Autodesk Inventor part; units mm, degrees
ref_plane "YZ Plane" through (0, 0, 0) normal (1, 0, 0) x (0, 1, 0)
ref_plane "XZ Plane" through (0, 0, 0) normal (0, 1, 0) x (-1, 0, 0)
ref_plane "XY Plane" through (0, 0, 0) normal (0, 0, 1) x (1, 0, 0)
sketch "Skizze1" plane through (0, 0, 0) normal (0, 1, 0) x (-1, 0, 0)
  line L0 (-20.5, 20.5) -> (20.5, 20.5)
  line L1 (20.5, 20.5) -> (20.5, -20.5)
  line L2 (20.5, -20.5) -> (-20.5, -20.5)
  line L3 (-20.5, -20.5) -> (-20.5, 20.5)
  line L4 (-20.5, 20.5) -> (20.5, -20.5) construction
  line L5 (20.5, 20.5) -> (-20.5, -20.5) construction
  point P0 (0, 0)
  dimension "d0" = 41
  dimension "d1" = 41
extrude "Extrusion1" add sketch "Skizze1" along normal mid plane 39
sketch "Skizze2" plane through (0, -19.5, 0) normal (0, -1, 0) x (1, 0, 0)
  line L0 (-20.5, 20.5) -> (20.5, 20.5)
  line L1 (-7.5, 20.5) -> (7.5, 20.5)
  line L2 (7.5, 20.5) -> (7.5, 23.5)
  line L3 (7.5, 23.5) -> (-7.5, 23.5)
  line L4 (-7.5, 23.5) -> (-7.5, 20.5)
  line L5 (0, -29.3) -> (0, 32.3)
  point P0 (0, 0)
  dimension "d4" = 15
  dimension "d5" = 3
extrude "Extrusion2" add sketch "Skizze2" against normal blind 3
sketch "Skizze3" plane through (0, -19.5, 0) normal (0, -1, 0) x (1, 0, 0)
  line L0 (-15.5, -15.5) -> (15.5, -15.5)
  line L1 (15.5, -15.5) -> (15.5, 15.5)
  line L2 (15.5, 15.5) -> (-15.5, 15.5)
  line L3 (-15.5, 15.5) -> (-15.5, -15.5)
  line L4 (-15.5, -15.5) -> (15.5, 15.5) construction
  line L5 (15.5, -15.5) -> (-15.5, 15.5) construction
  circle A0 centre (-15.5, 15.5) radius 1.5
  circle A1 centre (15.5, 15.5) radius 1.5
  circle A2 centre (15.5, -15.5) radius 1.5
  circle A3 centre (-15.5, -15.5) radius 1.5
  circle A4 centre (0, 0) radius 4.5
  dimension "d8" = 31
  dimension "d9" = 31
  dimension "d10" = 3
  dimension "d11" = 9
extrude "Extrusion3" cut sketch "Skizze3" along normal through all both and the other way through all contours L3 A3 L0 | L0 A3 L3 | A2 L1 L0 | L0 L1 A2 | A0 L2 L3 | L3 L2 A0 | A1 L2 L1 | L1 L2 A1 | A4
chamfer "Fase1" distance 4 angle 45 4 edges at (20.5, 0, 20.5) (-20.5, 0, 20.5) (20.5, 0, -20.5) (-20.5, 0, -20.5)
sketch "Skizze4" plane through (0, 0, 0) normal (0, 1, 0) x (-1, 0, 0)
  line L0 (19.5, 14.6716) -> (14.6716, 19.5)
  line L1 (-14.6716, 19.5) -> (-19.5, 14.6716)
  line L2 (-19.5, -14.6716) -> (-14.6716, -19.5)
  line L3 (14.6716, -19.5) -> (19.5, -14.6716)
  line L4 (25.5, -25.5) -> (-25.5, -25.5)
  line L5 (-25.5, -25.5) -> (-25.5, 25.5)
  line L6 (-25.5, 25.5) -> (25.5, 25.5)
  line L7 (25.5, 25.5) -> (25.5, -25.5)
  line L8 (25.5, -25.5) -> (-25.5, 25.5) construction
  line L9 (-25.5, -25.5) -> (25.5, 25.5) construction
  line L10 (-20.5, 16.5) -> (-16.5, 20.5)
  line L11 (-16.5, -20.5) -> (-20.5, -16.5)
  line L12 (20.5, -16.5) -> (16.5, -20.5)
  line L13 (16.5, 20.5) -> (20.5, 16.5)
  line L14 (19.5, 14.6716) -> (19.5, -14.6716)
  line L15 (14.6716, -19.5) -> (-14.6716, -19.5)
  line L16 (-19.5, -14.6716) -> (-19.5, 14.6716)
  line L17 (-14.6716, 19.5) -> (14.6716, 19.5)
  line L18 (16.5, 20.5) -> (-16.5, 20.5)
  line L19 (-20.5, 16.5) -> (-20.5, -16.5)
  line L20 (-16.5, -20.5) -> (16.5, -20.5)
  line L21 (20.5, -16.5) -> (20.5, 16.5)
  point P0 (0, 0)
  dimension "d21" = 2
  dimension "d22" = 1
  dimension "d24" = 1
  dimension "d25" = 1
extrude "Extrusion4" cut sketch "Skizze4" along normal mid plane 22 contours L4 L5 L6 L7 | L10 L18 L13 L21 L12 L20 L11 L19
sketch "Skizze6" plane through (-7.5, -16.5, 20.5) normal (0, 0, 1) x (1, 0, 0)
  line L0 (0, 0) -> (15, 0)
  line L1 (15, 0) -> (15, 3)
  line L2 (15, 3) -> (0, 3)
  line L3 (0, 3) -> (0, 0)
  line L4 (15, -3) -> (15, 0)
  line L5 (0, -3) -> (0, 0)
  line L6 (0, 0) -> (15, 0)
  line L7 (2.5, 1) -> (3.5, 1)
  line L8 (3.5, 1) -> (3.5, 2)
  line L9 (3.5, 2) -> (2.5, 2)
  line L10 (2.5, 2) -> (2.5, 1)
  line L11 (2.5, 1) -> (3.5, 2) construction
  line L12 (3.5, 1) -> (2.5, 2) construction
  line L13 (5.5, 1) -> (6.5, 1)
  line L14 (6.5, 1) -> (6.5, 2)
  line L15 (6.5, 2) -> (5.5, 2)
  line L16 (5.5, 2) -> (5.5, 1)
  line L17 (5.5, 1) -> (6.5, 2) construction
  line L18 (6.5, 1) -> (5.5, 2) construction
  line L19 (8.5, 1) -> (9.5, 1)
  line L20 (9.5, 1) -> (9.5, 2)
  line L21 (9.5, 2) -> (8.5, 2)
  line L22 (8.5, 2) -> (8.5, 1)
  line L23 (8.5, 1) -> (9.5, 2) construction
  line L24 (9.5, 1) -> (8.5, 2) construction
  line L25 (11.5, 1) -> (12.5, 1)
  line L26 (12.5, 1) -> (12.5, 2)
  line L27 (12.5, 2) -> (11.5, 2)
  line L28 (11.5, 2) -> (11.5, 1)
  line L29 (11.5, 1) -> (12.5, 2) construction
  line L30 (12.5, 1) -> (11.5, 2) construction
  line L31 (7.5, -10.8) -> (7.5, 43.8)
  point P0 (7.5, 16.5)
  point P1 (3, 1.5)
  point P2 (6, 1.5)
  point P3 (9, 1.5)
  point P4 (12, 1.5)
  point P5 (12, 1.5)
  point P6 (15, 1.5)
  dimension "d29" = 3
  dimension "d30" = 3
  dimension "d31" = 3
  dimension "d32" = 1
  dimension "d33" = 1
extrude "Extrusion6" cut sketch "Skizze6" against normal blind 5
sketch "Skizze7" plane through (0, 0, 0) normal (1, 0, 0) x (0, 1, 0)
  line L0 (34.5, 0) -> (34.5, 2.5)
  line L1 (34.5, 2.5) -> (20.5, 2.5)
  line L2 (20.5, 2.5) -> (20.5, 7.5)
  line L3 (20.5, 7.5) -> (19.5, 7.5)
  line L4 (19.5, -16.5) -> (19.5, 16.5)
  line L5 (19.5, 0) -> (34.5, 0)
  line L6 (19.5, 0) -> (19.5, 7.5)
  line L7 (38.5419, 0) -> (33.7383, 0)
  point P0 (0, 0)
  dimension "d37" = 5
  dimension "d38" = 1
  dimension "d39" = 15
  dimension "d40" = 15
revolve "Umdrehung1" add sketch "Skizze7" angle 360 about axis through (0, 19.5, 0) along (0, 1, 0)
equation "\"d24\" = d22"
equation "\"d25\" = d22"
equation "\"d33\" = d32"
properties part number "MotorBlock"
Source: CAD feature listing. Evaluate the final solid. Frame: model axes, mm. A direction names the side the tool comes from. Round coordinates to 2 decimals unless told otherwise and drop trailing zeros. Loops run counter-clockwise (first coordinate to the right, second up) from the corner with the lowest first, then second, coordinate; pieces in that order, holes last. Notation, with made-up numbers: M 23.5,83 L 27.5,83 A7 ccw 27.5,94 Z; hole C -34.75,37 d4. An arc over 180 degrees is marked long. Use a Markdown table: item, result. Add a question column.
1. Contact query for flat-ended pins moving along their axis: pin 1 (9.5 mm diameter, centred on x = 5, y = 17, fed in from +Z); pin 2 (1.5 mm diameter, centred on y = -18, z = 22.5, fed in from +X); pin 3 (1.5 mm diameter, centred on y = 20.5, z = -12.5, fed in from +X); pin 4 (1.5 mm diameter, centred on x = 13.5, y = 3.5, fed in from -Z). Output: stop coordinate, or through.
2. Cut plane B-B, the plane x = -10. Output: boundary loops of the cut face in (y, z), and give its area (4 significant figures).
3. Cut plane A-A, the plane y = 16.5. Output: boundary loops of the cut face in (x, z).
4. Cut plane C-C, the plane z = -8.5. Output: boundary loops of the cut face in (x, y), and give its area (4 significant figures).
5. Ray query, line 1 along Y through (x, z) = (-7, 20); line 2 along Z through (x, y) = (-15, 10); line 3 along Z through (x, y) = (0, -9.5). Return the intervals inside material, ascending. Write a range as [from, to].
6. Set-up query: faces 1 (the flat face through (17.12, 0.15, -17.05)), 2 (the flat face through (-17.05, 0.15, -17.12)), 3 (the flat face through (2, 20.5, -2)), 4 (the flat face through (0, -13.5, 18)), 5 (the flat face through (0, 0, 19.5)). Return all of +Z, -Z, +X, -X, +Y, -Y with unobstructed straight access to the full face (end or side cutting, diameter ignored); none if empty.
7. Pull-direction query (X, two-part tool) for faces 6 (the flat face through (0, 19.5, -9)), 7 (the flat face through (-7.5, -18, 22)), 8 (the flat face through (20.5, -15, 0)), 9 (the flat face through (7.5, -15, 18)); classes: +X half, -X half, draft (parallel to the pull), parting line (faces both ways), or undercut.
8. Cut plane D-D, the plane x = -15.5. Output: boundary loops of the cut face in (y, z), and give its area (3 significant figures).
Solution:
| question | item | result |
|---|---|---|
| 1 | pin 1 | stops at z = 20.5 |
| 1 | pin 2 | stops at x = 7.5 |
| 1 | pin 3 | passes through |
| 1 | pin 4 | stops at z = -19.5 |
| 2 | outline | M -19.5,-20.5 L -11,-20.5 L -11,-19.5 L 11,-19.5 L 11,-20.5 L 19.5,-20.5 L 19.5,20.5 L 11,20.5 L 11,19.5 L -11,19.5 L -11,20.5 L -19.5,20.5 Z |
| 2 | area | 1,555 mm2 |
| 3 | outline | M -20.5,-16.5 L -16.5,-20.5 L 16.5,-20.5 L 20.5,-16.5 L 20.5,16.5 L 16.5,20.5 L -16.5,20.5 L -20.5,16.5 Z; hole C -15.5,-15.5 d3; hole C -15.5,15.5 d3; hole C 0,0 d9; hole C 15.5,-15.5 d3; hole C 15.5,15.5 d3 |
| 4 | outline | M -20.5,-19.5 L 20.5,-19.5 L 20.5,-11 L 19.5,-11 L 19.5,11 L 20.5,11 L 20.5,19.5 L -20.5,19.5 L -20.5,11 L -19.5,11 L -19.5,-11 L -20.5,-11 Z |
| 4 | area | 1,555 mm2 |
| 5 | line 1 | y = [-19.5, -16.5], [-13.5, -11], [11, 19.5] |
| 5 | line 2 | z = [-19.17, -16.91], [-14.09, 14.09], [16.91, 19.17] |
| 5 | line 3 | z = [-19.5, -4.5], [4.5, 19.5] |
| 6 | face 1 | -Z, +X |
| 6 | face 2 | -Z, -X |
| 6 | face 3 | +Y |
| 6 | face 4 | +Z |
| 6 | face 5 | +Z, +X, -X |
| 7 | face 6 | draft |
| 7 | face 7 | -X half |
| 7 | face 8 | +X half |
| 7 | face 9 | undercut |
| 8 | outline | M -19.5,-20.5 L -11,-20.5 L -11,-18.67 L 11,-18.67 L 11,-20.5 L 19.5,-20.5 L 19.5,-17 L -19.5,-17 Z; M -19.5,-14 L 19.5,-14 L 19.5,14 L -19.5,14 Z; M -19.5,17 L 19.5,17 L 19.5,20.5 L 11,20.5 L 11,18.67 L -11,18.67 L -11,20.5 L -19.5,20.5 Z |
| 8 | area | 1,280 mm2 |
